Read the model definition and answer for the solid it produces. Units are mm, in the model's axes. Face numbers are marked on the shaded views. Coordinates: 2 decimals unless noted, no trailing zeros. Order: outer loops, then holes, each group sorted by start corner. A loop starts at its lowest first (then second) coordinate and runs counter-clockwise, first axis right, second up. Notation, with made-up numbers: M -5.75,51 L 6.25,51 A16 cw 6.25,74 Z; hole C 20.5,76 d7. An arc over 180 degrees is marked long. One line per question, with ' | ' between items. Start each with the question number.
1) Find section B-B, the plane z = 1.5. Write down the section's boundary in (x, y) (3 decimals).
2) Find section D-D, the plane x = -5.5. Write down the section's boundary in (y, z), plus the area to 3 significant figures.
3) The mould has two halves that part along Y. Classify the marked faces 1, 2 and 3: +Y half, -Y half, draft (parallel to the pull), parting line (faces both ways), or undercut.
4) Consider probe 1 along Y at (x, z) = (-3.5, 1.5); probe 2 along X at (y, z) = (36, 1.5); probe 3 along Y at (x, z) = (-5.75, 3.75). Determine where each line is inside the solid, lowest interval first.
5) Find section C-C, the plane y = 38.5. Write down the section's boundary in (x, z), plus the area to 3 significant figures.
6) Given P1, Ø1.5, axis at y = 21, z = 4, coming from the -X side; P2, Ø1.5, axis at y = 26.5, z = 1, coming from the +X side, each flat-ended and moving along its own axis, determine where each tip first touches the part or whether it passes through.
7) Find section A-A, the plane x = 4. Write down the section's boundary in (y, z).
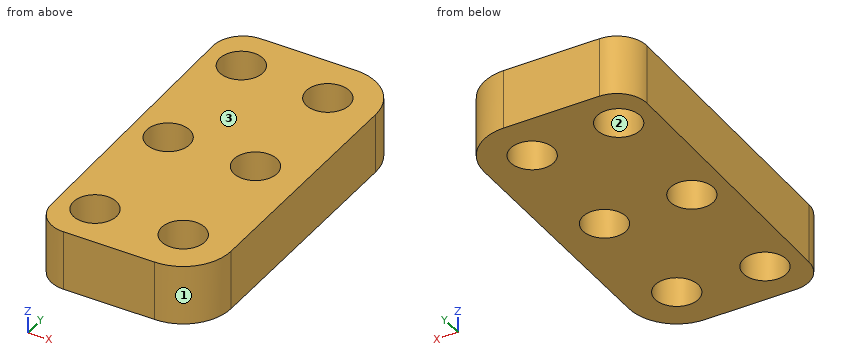
Autodesk Inventor part; units mm, degrees
ref_plane "Work Plane1" through (0.394452, -0.667998, 0) normal (0, 0, 1) x (0.9998788, 0.0155691, 0)
ref_plane "YZ Plane" through (0, 0, 0) normal (1, 0, 0) x (0, 1, 0)
ref_plane "XZ Plane" through (0, 0, 0) normal (0, 1, 0) x (-1, 0, 0)
ref_plane "Work Plane1" through (0.394452, -0.667998, 0) normal (0, 0, 1) x (0.9998788, 0.0155691, 0)
sketch "Sketch1" plane through (0.394452, -0.667998, 0) normal (0, 0, 1) x (0.9998788, 0.0155691, 0)
  circle A0 centre (5.204347, 38.285312) radius 1.27
  circle A1 centre (5.004519, 25.586884) radius 1.27
  circle A2 centre (4.796193, 12.888588) radius 1.27
  line L0 (5.002396, 38.285413) -> (4.989697, 12.888491) construction
  line L1 (0.125003, 38.366943) -> (-0.283151, 12.970219)
  line L2 (9.875538, 12.806957) -> (10.283691, 38.203681)
  arc A3 (10.283691, 38.203681) -> (0.125003, 38.366943) centre (5.204347, 38.285312) ccw
  arc A4 (-0.283151, 12.970219) -> (9.875538, 12.806957) centre (4.796193, 12.888588) ccw
  circle A5 centre (4.796193, 12.888588) radius 2.286
  circle A6 centre (4.996047, 25.587018) radius 2.286
  circle A7 centre (5.204347, 38.285312) radius 2.286
  line L3 (4.714563, 7.809244) -> (-4.810437, 7.809244)
  line L4 (-7.985437, 10.984244) -> (-7.985437, 40.194244)
  line L5 (-4.808994, 43.369244) -> (5.285978, 43.364656)
  arc A8 (-7.985437, 10.984244) -> (-4.810437, 7.809244) centre (-4.810437, 10.984244) ccw
  arc A9 (-4.808994, 43.369244) -> (-7.985437, 40.194244) centre (-4.810437, 40.194244) ccw
  circle A10 centre (-4.175437, 12.381244) radius 2.286
  circle A11 centre (-4.175437, 25.586884) radius 2.286
  circle A12 centre (-4.175437, 38.796956) radius 2.286
  point P0 (-0.384004, 0.674059)
  point P1 (-7.985437, 7.809244)
  dimension "d0" = 10.16
  dimension "d1" = 4.572
  dimension "d2" = 4.572
  dimension "d3" = 4.572
  dimension "d4" = 12.7
  dimension "d6" = 3.175
  dimension "d7" = 3.175
  dimension "d8" = 35.56
  dimension "d18" = 3.81
  dimension "d19" = 4.572
  dimension "d20" = 4.572
  dimension "d21" = 4.572
sketch "Sketch1 outline for Extrusion1" plane through (0.394452, -0.667998, 0) normal (0, 0, 1) x (0.9998788, 0.0155691, 0)
  line L0 (5.285978, 43.364656) -> (-4.808994, 43.369244)
  arc A0 (10.283691, 38.203681) -> (5.285978, 43.364656) centre (5.204347, 38.285312) ccw
  arc A1 (-4.808994, 43.369244) -> (-7.985437, 40.194244) centre (-4.810437, 40.194244) ccw
  line L1 (9.875538, 12.806957) -> (10.283691, 38.203681)
  line L2 (-7.985437, 40.194244) -> (-7.985437, 10.984244)
  arc A2 (4.714563, 7.809244) -> (9.875538, 12.806957) centre (4.796193, 12.888588) ccw
  arc A3 (-7.985437, 10.984244) -> (-4.810437, 7.809244) centre (-4.810437, 10.984244) ccw
  line L3 (-4.810437, 7.809244) -> (4.714563, 7.809244)
  circle A4 centre (-4.175437, 12.381244) radius 2.286
  circle A5 centre (-4.175437, 25.586884) radius 2.286
  circle A6 centre (4.796193, 12.888588) radius 2.286
  circle A7 centre (4.996047, 25.587018) radius 2.286
  circle A8 centre (-4.175437, 38.796956) radius 2.286
  circle A9 centre (5.204347, 38.285312) radius 2.286
extrude "Extrusion1" add sketch "Sketch1 outline for Extrusion1" along normal blind 6.35
properties part number "OdomPods" material "Plastic, Opaque Black"
Report:
1) outline: M -8.216,39.397 L -7.761,10.191 A3.175 ccw -4.537,7.065 L 4.987,7.214 A5.08 ccw 10.069,12.291 L 10.082,37.691 A5.08 ccw 5.005,42.774 L -5.089,42.621 A3.175 ccw Z; hole C -4.385,38.059 d4.572; hole C -4.179,24.851 d4.572; hole C -3.973,11.647 d4.572; hole C 4.989,12.294 d4.572; hole C 4.992,24.994 d4.572; hole C 5.002,37.694 d4.572
2) outline: M 7.2,0 L 9.95,0 L 9.95,6.35 L 7.2,6.35 Z; M 13.35,0 L 22.99,0 L 22.99,6.35 L 13.35,6.35 Z; M 26.72,0 L 36.06,0 L 36.06,6.35 L 26.72,6.35 Z; M 40.05,0 L 42.59,0 L 42.59,6.35 L 40.05,6.35 Z | area: 154 mm^2
3) face 1: -Y half | face 2: undercut | face 3: draft
4) probe 1: y = 7.08 to 9.41, 13.88 to 22.67, 27.03 to 35.95, 40.17 to 42.65 | probe 2: x = -8.16 to -5.38, -3.39 to 3.47, 6.54 to 10.08 | probe 3: y = 7.29 to 10.21, 13.09 to 23.19, 26.51 to 36.23, 39.89 to 42.54
5) outline: M -8.2,0 L -6.63,0 L -6.63,6.35 L -8.2,6.35 Z; M -2.14,0 L 2.86,0 L 2.86,6.35 L -2.14,6.35 Z; M 7.14,0 L 10.02,0 L 10.02,6.35 L 7.14,6.35 Z | area: 60.0 mm^2
6) P1: stops at x = -7.94 | P2: stops at x = 10.08
7) outline: M 7.2,0 L 10.23,0 L 10.23,6.35 L 7.2,6.35 Z; M 14.35,0 L 22.93,0 L 22.93,6.35 L 14.35,6.35 Z; M 27.05,0 L 35.64,0 L 35.64,6.35 L 27.05,6.35 Z; M 39.75,0 L 42.76,0 L 42.76,6.35 L 39.75,6.35 Z
